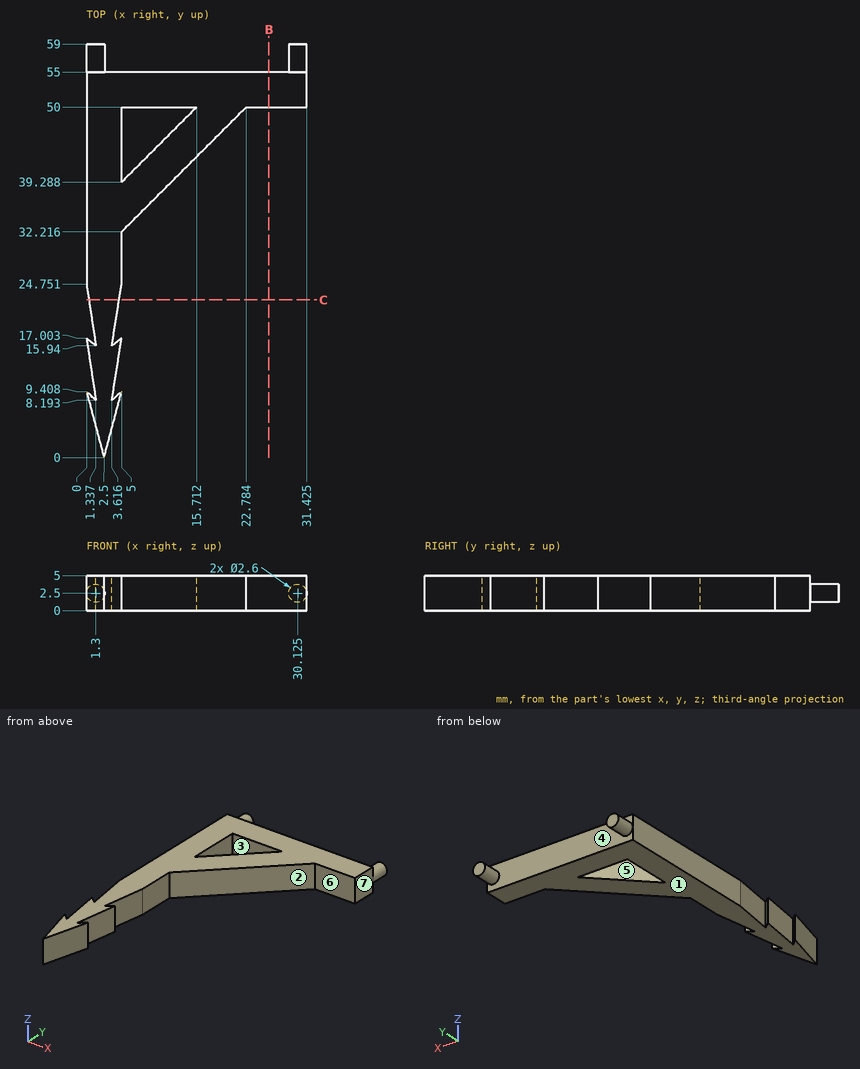
The figure shows three views and two pictorial views of one solid part (mm, origin at its lowest corner). Answer the questions. A direction names the side the tool comes from. Round coordinates to 2 decimals unless told otherwise and drop trailing zeros. Write each loop counter-clockwise with the first axis right and the second up, starting at its lowest first coordinate (ties: lowest second). Pieces come first, ordered by that corner, then holes. Notation, with made-up numbers: M 12.25,40 L 48.25,40 A12 cw 48.25,54 Z; hole C 6.25,73.25 d9. An arc over 180 degrees is marked long. Write each question's results on one line, items separated by ' | '. Start each with the question number.
(1) Find the intervals of material crossed by line 1 (Y direction, x = 23, z = 4.7); line 2 (X direction, y = 41, z = 2.5) (1 decimal); line 3 (Y direction, x = 12.5, z = 2.05) (1 decimal), in increasing order.
(2) Determine the mould class of the marked faces 1, 2, 3 and 4 for opening direction Y: +Y half, -Y half, draft (parallel to the pull), parting line (faces both ways), or undercut.
(3) For the marked faces 5, 6 and 7, determine the directions among +Z, -Z, +X, -X, +Y, -Y from which every point of the face is accessible in a straight line to the end or side of a thin tool.
(4) The part is cut by section B-B, the plane x = 26. Write down the section's boundary in (y, z), and give its area (3 significant figures).
(5) Each of these flat-tipped pins is pushed along its axis until it touches: P1, Ø2.5, axis at y = 47, z = 3.5, coming from the +X side (1 decimal); P2, Ø1.5, axis at y = 33, z = 4, coming from the +X side (1 decimal); P3, Ø1.5, axis at y = 28.5, z = 1.5, coming from the +X side. Where does it stop, or does it pass through?
(6) The part is cut by section C-C, the plane y = 22.5. Write down the section's boundary in (x, z), and give its area (3 significant figures).
Worked answers:
1) line 1: y = 50 to 55 | line 2: x = 0 to 5, 6.7 to 13.8 | line 3: y = 39.7 to 46.8, 50 to 55
2) face 1: draft | face 2: -Y half | face 3: undercut | face 4: +Y half
3) face 5: +Z, -Z | face 6: +Z, -Z, +X, -Y | face 7: +Z, -Z, +X, +Y, -Y
4) outline: M 50,0 L 55,0 L 55,5 L 50,5 Z | area: 25.0 mm²
5) P1: stops at x = 21 | P2: stops at x = 6.5 | P3: stops at x = 5
6) outline: M 0.34,0 L 4.65,0 L 4.65,5 L 0.34,5 Z | area: 21.5 mm²
